from build123d import *

# Parameters (mm, degrees)
F2_R = 9.525
F3_R = 5.08


with BuildPart() as f1:
    # F0 (on Front) → F1 (revolve)
    with BuildSketch(Plane.XZ):
        with BuildLine():
            Line((0, 2.54), (0, 0))
            Line((0, 0), (26.162, 0))
            Line((26.162, 0), (23.063575, 59.121467))
            ThreePointArc((23.063575, 59.121467), (21.728849, 60.32326), (20.527056, 58.988533))
            Line((20.527056, 58.988533), (23.485398, 2.54))
            Line((23.485398, 2.54), (0, 2.54))
        make_face()
    revolve(axis=Axis((0, 0, 30.1625), (0, 0, 1)))

    # F2
    f2_edges = [f1.edges().sort_by_distance(p)[0] for p in [
        (-23.485398, 0, 2.54),
    ]]
    fillet(f2_edges, radius=F2_R)

    # F3
    f3_edges = [f1.edges().sort_by_distance(p)[0] for p in [
        (-26.162, 0, 0),
    ]]
    fillet(f3_edges, radius=F3_R)


solid = f1.part
Geometry check sheet. Reference: the model listing, model coordinates, mm. Coordinates: 2 decimals unless noted, no trailing zeros. Order: outer loops, then holes, each group sorted by start corner. A loop starts at its lowest first (then second) coordinate and runs counter-clockwise, first axis right, second up. Notation, with made-up numbers: M 34.5,23 L 74.5,23 A24 ccw 74.5,33 Z; hole C 51.25,19.25 d5. An arc over 180 degrees is marked long. Use CSV: the item, a comma, the result in double quotes.
Item 1: Cross-section at C-C on z = 38. Record the cut outline in (x, y), then the cut area to 3 significant figures.
Returned:
outline,"C 0,0 d48.34; hole C 0,0 d43.25"
area,"366 mm2"
Item 2: Thickness scan on line 1 along Z through (x, y) = (9, -3); line 2 along X through (y, z) = (18.5, 11); line 3 along X through (y, z) = (-18, 25.5). Record the ranges inside material, lowest first.
Returned:
line 1,"z = 0 to 2.54"
line 2,"x = -17.67 to -13.52, 13.52 to 17.67"
line 3,"x = -17.1 to -13.13, 13.13 to 17.1"
Item 3: Cross-section at D-D on z = 48. Record the cut outline in (x, y).
Returned:
outline,"C 0,0 d47.29; hole C 0,0 d42.21"
Item 4: Mould release check, pull along X, two halves, no side actions. Record for faces 1 (the flat face through (0, 0, 0)), 2 (the flat face through (0, 0, 2.54)), 3 (the conical face through (-19.405, -14.879, 32.61)): pulls with the +X half, pulls with the -X half, needs draft (parallel to the pull), parting line crosses it, or undercut.
Returned:
face 1,"needs draft"
face 2,"undercut"
face 3,"parting line crosses it"
Item 5: Gauge pin test, flat ends, axial feed: pin 1 Ø21.5 at (x, y) = (0.5, 1.5) entering from +Z; pin 2 Ø8 at (y, z) = (-8.5, 27.5) entering from +X; pin 3 Ø6 at (y, z) = (-12, 48) entering from -X; pin 4 Ø3 at (x, y) = (5, 12.5) entering from -Z. Record the tip position at first contact, or that the pin passes through.
Returned:
pin 1,"stops at z = 2.54"
pin 2,"stops at x = 24.34"
pin 3,"stops at x = -21.88"
pin 4,"stops at z = 0"
